Autodesk Inventor part; units mm, degrees
ref_plane "YZ Plane" through (0, 0, 0) normal (1, 0, 0) x (0, 1, 0)
ref_plane "XZ Plane" through (0, 0, 0) normal (0, 1, 0) x (-1, 0, 0)
ref_plane "XY Plane" through (0, 0, 0) normal (0, 0, 1) x (1, 0, 0)
sketch "Profile" plane through (0, 0, 0) normal (0, 0, 1) x (1, 0, 0)
  line L0 (-18, 0) -> (-18, 11)
  line L1 (-18, 11) -> (0, 11)
  line L2 (0, 11) -> (0.5774, 12)
  line L3 (0.5774, 12) -> (38.0774, 12)
  line L4 (38.0774, 12) -> (38.6547, 11)
  line L5 (38.6547, 11) -> (57, 11)
  line L6 (57, 11) -> (57, 0)
  line L7 (-18, 0) -> (0, 0)
  line L8 (0, 0) -> (0, 9)
  line L9 (0, 9) -> (49, 9)
  line L10 (49, 9) -> (49, 0)
  line L11 (49, 0) -> (57, 0)
  line L12 (-33, 0) -> (72, 0) construction
  line L13 (0, 11) -> (0, 9) construction
  dimension "BodyLength" = 75
  dimension "d1" = 11
  dimension "d3" = 120
  dimension "d4" = 120
  dimension "d5" = 37.5
  dimension "d6" = 18
  dimension "d16" = 8
  dimension "d29" = 1
  dimension "d30" = 9
revolve "ProfileRevolveFeature" add sketch "Profile" angle 360 about axis through (-10, 0, 0) along (1, 0, 0)
sketch "InsideHole" plane through (-18, 0, 0) normal (-1, 0, 0) x (0, 0, 1)
  circle A0 centre (0, 0) radius 9 construction
hole "InsideHoleFeature" at (-18, 0, 0) direction (1, 0, 0) diameter 19 end through all
chamfer "EndChamferFeature" distance 1 angle 45 1 edges at (-18, -11, 0)
sketch "CapMountHole" plane through (0, 0, 0) normal (0, 1, 0) x (-1, 0, 0)
  line L0 (-57, 11) -> (-57, -11) construction
  line L1 (14.44, 0) -> (-86.64, 0) construction
  circle A0 centre (-52.5, 0) radius 1.25
  point P0 (0, 0)
  dimension "d31" = 4.5
  dimension "d39" = 2.5
extrude "CapMountHoleFeature" cut sketch "CapMountHole" along normal through all both and the other way through all
equation "\"d5\" = 0.5 * BodyLength"
equation "\"d6\" = 0.24 * BodyLength"
properties part number "BackPair1PistonBody"
Source: CAD feature listing. Evaluate the final solid. Frame: model axes, mm. A direction names the side the tool comes from. Coordinates: 2 decimals unless noted, no trailing zeros. Write each loop counter-clockwise with the first axis right and the second up, starting at its lowest first coordinate (ties: lowest second). Pieces come first, ordered by that corner, then holes. Notation, with made-up numbers: (-2, -33) -> (26, -33) arc R27 ccw to (26, -4) -> close; hole circle Ø6 at (51, 56). An arc over 180 degrees is marked (long way). Return JSON: item names as keys, results as strings. Group by question number.
1) Contact query for flat-ended pins moving along their axis: P1, Ø6, axis at x = 24, y = 3.5, coming from the +Z side; P2, Ø6, axis at x = 30.5, z = 1, coming from the -Y side; P3, Ø1, axis at x = 39, y = 1, coming from the -Z side; P4, Ø6, axis at x = 39.5, z = -9, coming from the -Y side. Output: stop coordinate, or through.
2) Section query A-A, the plane y = 0. Return loops of the section in (x, z).
3) Section query D-D, the plane x = 52.5. Return loops of the section in (y, z).
4) Ray query, line 1 along Z through (x, y) = (-1, 0); line 2 along Z through (x, y) = (36, 0); line 3 along Y through (x, z) = (40, -7). Return the intervals inside material, ascending.
5) Mould query, pull axis Z, two halves, no side actions, for faces 4 (the face through (57, -10, 0)), 5 (the face through (51.31, -10.2, 0.38)), 6 (the face through (51.31, 10.2, -0.38)), 7 (the face through (19.59, -11.99, 0.53)). Classes: +Z half, -Z half, draft (parallel to the pull), parting line (faces both ways), or undercut.
6) Set-up query: faces 1 (the face through (47.956, 10.161, -4.213)), 2 (the face through (-8.38, -2.38, -10.74)), 3 (the face through (-18, 9, -4)). Return all of +Z, -Z, +X, -X, +Y, -Y with unobstructed straight access to the full face (end or side cutting, diameter ignored); none if empty.
7) Section query C-C, the plane x = -10. Return loops of the section in (y, z).
8) Section query B-B, the plane z = 0. Return loops of the section in (x, y).
From the geometry:
{
 "1": {"P1": "z = 11.99", "P2": "y = -12", "P3": "z = -11.22", "P4": "y = -10.18"},
 "2": {"outline": "(-18, -10) -> (-17, -11) -> (0, -11) -> (0.58, -12) -> (38.08, -12) -> (38.65, -11) -> (57, -11) -> (57, -9.5) -> (-18, -9.5) -> close; (-18, 9.5) -> (57, 9.5) -> (57, 11) -> (38.65, 11) -> (38.08, 12) -> (0.58, 12) -> (0, 11) -> (-17, 11) -> (-18, 10) -> close"},
 "3": {"outline": "(-10.93, -1.25) arc R11 ccw to (10.93, -1.25) -> (9.42, -1.25) arc R9.5 cw to (-9.42, -1.25) -> close; (-10.93, 1.25) -> (-9.42, 1.25) arc R9.5 cw to (9.42, 1.25) -> (10.93, 1.25) arc R11 ccw to start"},
 "4": {"line 1": "-11 to -9.5, 9.5 to 11", "line 2": "-12 to -9.5, 9.5 to 12", "line 3": "-8.49 to -6.42, 6.42 to 8.49"},
 "5": {"face 4": "draft", "face 5": "undercut", "face 6": "undercut", "face 7": "parting line"},
 "6": {"face 1": "+X", "face 2": "-X", "face 3": "+Z, -Z, -X, +Y, -Y"},
 "7": {"outline": "circle Ø22 at (0, 0); hole circle Ø19 at (0, 0)"},
 "8": {"outline": "(-18, -10) -> (-17, -11) -> (0, -11) -> (0.58, -12) -> (38.08, -12) -> (38.65, -11) -> (51.25, -11) -> (51.25, -9.5) -> (-18, -9.5) -> close; (-18, 9.5) -> (51.25, 9.5) -> (51.25, 11) -> (38.65, 11) -> (38.08, 12) -> (0.58, 12) -> (0, 11) -> (-17, 11) -> (-18, 10) -> close; (53.75, -11) -> (57, -11) -> (57, -9.5) -> (53.75, -9.5) -> close; (53.75, 9.5) -> (57, 9.5) -> (57, 11) -> (53.75, 11) -> close"}
}
